Solid Edge part; units mm, degrees
sketch "Sketch1" plane through (0, 0, 0) normal (0, 0, 1) x (1, 0, 0)
  line L0 (139.7106, 161.4953) -> (139.7106, 27.4953)
  line L1 (139.7106, 27.4953) -> (306.7106, 27.4953)
  line L2 (306.7106, 27.4953) -> (306.7106, 161.4953)
  line L3 (139.7106, 161.4953) -> (306.7106, 161.4953)
  dimension "D1" = 139.7106
  dimension "D2" = 139.7106
  dimension "D3" = 306.7106
extrude "Protrusion1" add sketch "Sketch1" against normal blind 47
sketch "Sketch2" plane through (223.2106, 94.4953, -47) normal (0, 0, -1) x (1, 0, 0)
  line L0 (83.5, 0) -> (83.5, 10.5)
  line L1 (83.5, 10.5) -> (-83.5, 10.5)
  line L2 (-83.5, 10.5) -> (-83.5, 0)
  line L3 (-83.5, 0) -> (-83.5, -10.5)
  line L4 (-83.5, -10.5) -> (83.5, -10.5)
  line L5 (83.5, 0) -> (83.5, -10.5)
  dimension "D1" = 83.5
  dimension "D2" = 83.5
  dimension "D3" = 83.5
extrude "ExtrudedCutout_1" cut sketch "Sketch2" against normal blind 20
sketch "Sketch3" plane through (223.2106, 94.4953, 0) normal (0, 0, 1) x (1, 0, 0)
  circle A0 centre (73.5, 0) radius 2.05
  circle A1 centre (64.5, 0) radius 2.05
  circle A2 centre (-17.5, 0) radius 2.05
  dimension "D1" = 73.5
extrude "Cutout1" cut sketch "Sketch3" against normal through all
sketch "Sketch4" plane through (223.2106, 94.4953, -27) normal (0, 0, -1) x (-1, 0, 0)
  line L0 (-78.5, 8) -> (-78.5, -8)
  line L1 (-78.5, -8) -> (24.5, -8)
  line L2 (24.5, 8) -> (24.5, -8)
  line L3 (-78.5, 8) -> (24.5, 8)
  dimension "D1" = 78.5
  dimension "D2" = 78.5
  dimension "D3" = 24.5
extrude "ExtrudedCutout_3" cut sketch "Sketch4" against normal blind 22
sketch "Sketch5" plane through (223.2106, 94.4953, 0) normal (0, 0, 1) x (0, 1, 0)
  circle A0 centre (0, 17.5) radius 62
extrude "ExtrudedCutout_4" cut sketch "Sketch5" against normal blind 5
chamfer "Chamfer_1" distance 1 angle 45 1 edges at (139.7106, 94.4953, 0)
chamfer "Chamfer_2" distance 1 angle 45 1 edges at (223.7106, 27.4953, 0)
chamfer "Chamfer_3" distance 1 angle 45 1 edges at (306.7106, 94.9953, 0)
chamfer "Chamfer_4" distance 1 angle 45 1 edges at (223.2106, 161.4953, 0)
sketch "Sketch6" plane through (223.2106, 94.4953, 0) normal (0, 0, 1) x (1, 0, 0)
  circle A0 centre (64.5, 0) radius 3.61
  circle A1 centre (73.5, 0) radius 3.61
extrude "ExtrudedCutout_5" cut sketch "Sketch6" against normal blind 4
sketch "Sketch7" plane through (306.7106, 94.4953, -24) normal (1, 0, 0) x (0, 1, 0)
  line L0 (8, -3) -> (8, 19)
  line L1 (28, 19) -> (8, 19)
  line L2 (28, -3) -> (28, 19)
  line L3 (8, -3) -> (28, -3)
  dimension "D1" = 8
extrude "ExtrudedCutout_6" cut sketch "Sketch7" against normal blind 30
sketch "Sketch8" plane through (223.2106, 55.7453, -47) normal (0, 0, -1) x (1, 0, 0)
  line L0 (-63.5, -8.25) -> (-43.5, -8.25)
  line L1 (-43.5, -8.25) -> (-43.5, -28.25)
  line L2 (-43.5, -28.25) -> (-63.5, -28.25)
  line L3 (-63.5, -28.25) -> (-63.5, -8.25)
  line L4 (-63.5, -69.25) -> (-43.5, -69.25)
  line L5 (-43.5, -69.25) -> (-43.5, -49.25)
  line L6 (-43.5, -49.25) -> (-63.5, -49.25)
  line L7 (-63.5, -69.25) -> (-63.5, -49.25)
  dimension "D1" = 63.5
  dimension "D2" = 63.5
  dimension "D3" = 63.5
extrude "ExtrudedCutout_9" cut sketch "Sketch8" against normal blind 20
sketch "Sketch9" plane through (223.2106, 55.7453, -47) normal (0, 0, -1) x (1, 0, 0)
  line L0 (43.5, -8.25) -> (63.5, -8.25)
  line L1 (63.5, -8.25) -> (63.5, -28.25)
  line L2 (43.5, -28.25) -> (63.5, -28.25)
  line L3 (43.5, -8.25) -> (43.5, -28.25)
  line L4 (43.5, -69.25) -> (63.5, -69.25)
  line L5 (63.5, -69.25) -> (63.5, -49.25)
  line L6 (43.5, -49.25) -> (63.5, -49.25)
  line L7 (43.5, -69.25) -> (43.5, -49.25)
  dimension "D1" = 43.5
  dimension "D2" = 43.5
extrude "ExtrudedCutout_10" cut sketch "Sketch9" against normal blind 20
sketch "Sketch10" plane through (223.2106, 27.4953, -24) normal (0, -1, 0) x (1, 0, 0)
  circle A0 centre (-53.5, -13) radius 2
extrude "Cutout2" cut sketch "Sketch10" against normal through all
sketch "Sketch11" plane through (223.2106, 27.4953, -24) normal (0, -1, 0) x (1, 0, 0)
  circle A0 centre (53.5, -13) radius 2
extrude "Cutout3" cut sketch "Sketch11" against normal through all
Verification items for the finished model (mm, model axes). A direction names the side the tool comes from. Coordinates: 2 decimals unless noted, no trailing zeros. Order: outer loops, then holes, each group sorted by start corner. A loop starts at its lowest first (then second) coordinate and runs counter-clockwise, first axis right, second up.
1. Sectioned sample at D-D, the plane x = 203. Record the cut outline in (y, z), and give its area (3 significant figures).
Results found:
outline: (27.5, -47) - (84, -47) - (84, -27) - (86.5, -27) - (86.5, -5) - (32.55, -5) - (32.55, 0) - (28.5, 0) - (27.5, -1) - close; (102.5, -27) - (105, -27) - (105, -47) - (161.5, -47) - (161.5, -1) - (160.5, 0) - (156.44, 0) - (156.44, -5) - (102.5, -5) - close
area: 4,910 mm2
2. Release check for a two-part mould opening along X. For faces 4 (the face through (276.711, 112, -16)), 5 (the face through (179.711, 74, -37)), 6 (the face through (277, 95, 0)) record: +X half, -X half, draft (parallel to the pull), parting line (faces both ways), or undercut.
Results found:
face 4: +X half
face 5: undercut
face 6: draft
3. Sectioned sample at C-C, the plane y = 47.5. Record the cut outline in (x, z), and give its area (3 significant figures).
Results found:
outline: (139.71, -47) - (306.71, -47) - (306.71, -1) - (305.71, 0) - (246.15, 0) - (246.15, -5) - (165.27, -5) - (165.27, 0) - (140.71, 0) - (139.71, -1) - close; hole circle Ø4 at (169.71, -37); hole circle Ø4 at (276.71, -37)
area: 7,420 mm2
4. Scan lines: line 1 (X direction, y = 78.5, z = -38.5); line 2 (Y direction, x = 244, z = -8); line 3 (X direction, y = 90.5, z = -19). Record each from-to range of solid material in increasing order.
Results found:
line 1: x = 139.71 to 159.71, 179.71 to 266.71, 286.71 to 306.71
line 2: y = 27.5 to 86.5, 102.5 to 161.5
line 3: x = 139.71 to 198.71, 301.71 to 306.71
5. Go/stop test with flat-tipped pins: pin 1 Ø1 at (x, y) = (233, 59) entering from +Z; pin 2 Ø10 at (y, z) = (116.5, -21.5) entering from +X. Record where each tip stops, or that it passes through.
Results found:
pin 1: stops at z = -5
pin 2: stops at x = 276.71
6. Set-up check for faces 1 (the face through (198.711, 95, -16)), 2 (the face through (284.846, 92.299, -1.972)), 3 (the face through (150, 83.995, -37)): record each of +Z, -Z, +X, -X, +Y, -Y from which the full face is reachable in a straight line by a thin tool's end or side.
Results found:
face 1: +Z, -Z
face 2: +Z
face 3: -Z, +X, -X
7. Sectioned sample at B-B, the plane z = -21.5. Record the cut outline in (x, y).
Results found:
outline: (139.71, 27.5) - (306.71, 27.5) - (306.71, 102.5) - (301.71, 102.5) - (301.71, 86.5) - (198.71, 86.5) - (198.71, 102.5) - (276.71, 102.5) - (276.71, 122.5) - (306.71, 122.5) - (306.71, 161.5) - (139.71, 161.5) - close
8. Sectioned sample at A-A, the plane x = 272.5. Record the cut outline in (y, z), and give its area (4 significant figures).
Results found:
outline: (27.5, -47) - (64, -47) - (64, -27) - (86.5, -27) - (86.5, -5) - (102.5, -5) - (102.5, -27) - (125, -27) - (125, -47) - (161.5, -47) - (161.5, -1) - (160.5, 0) - (28.5, 0) - (27.5, -1) - close
area: 4,725 mm2
